Verification items for this drawing (mm, ordinates from the low corner). A direction names the side the tool comes from. Round coordinates to 2 decimals unless told otherwise and drop trailing zeros. Loops run counter-clockwise (first coordinate to the right, second up) from the corner with the lowest first, then second, coordinate; pieces in that order, holes last. Notation, with made-up numbers: M 52.25,18.25 L 74.25,18.25 A15 cw 74.25,45.25 Z; hole C -39.75,5.5 d3. An arc over 180 degrees is marked long. Use one line per item in the form item = value. Start each with the question number.
1. Go/stop test with flat-tipped pins: pin 1 (1 mm diameter, centred on x = 10.5, y = 68, fed in from -Z); pin 2 (4.5 mm diameter, centred on x = 16, y = 12.5, fed in from +Z); pin 3 (8 mm diameter, centred on x = 3.5, y = 33, fed in from -Z); pin 4 (8 mm diameter, centred on y = 22.5, z = 19, fed in from -X). Record where each tip stops, or that it passes through.
2. Cross-section at A-A (y = 13.3). Record the boundary of the cut face in (x, z).
3. Draft check along Y on the marked faces 1, 2, 3 and 4. Enter one of: pulls with the +Y half, pulls with the -Y half, needs draft (parallel to the pull), parting line crosses it, or undercut.
4. Cross-section at D-D (x = 2.5). Record the boundary of the cut face in (y, z), then the cut area to 3 significant figures.
5. Set-up check for the marked faces 5, 6 and 7: record each of +Z, -Z, +X, -X, +Y, -Y from which the full face is reachable in a straight line by a thin tool's end or side.
6. Material ranges on line 1 (Y direction, x = 15, z = 33); line 2 (Y direction, x = 15, z = 48); line 3 (X direction, y = 13, z = 9), recorded low to high.
7. Cross-section at B-B (x = 15). Record the boundary of the cut face in (y, z), then the cut area to 3 significant figures.
8. Cross-section at C-C (z = 7). Record the boundary of the cut face in (x, y), then the cut area to 3 significant figures.
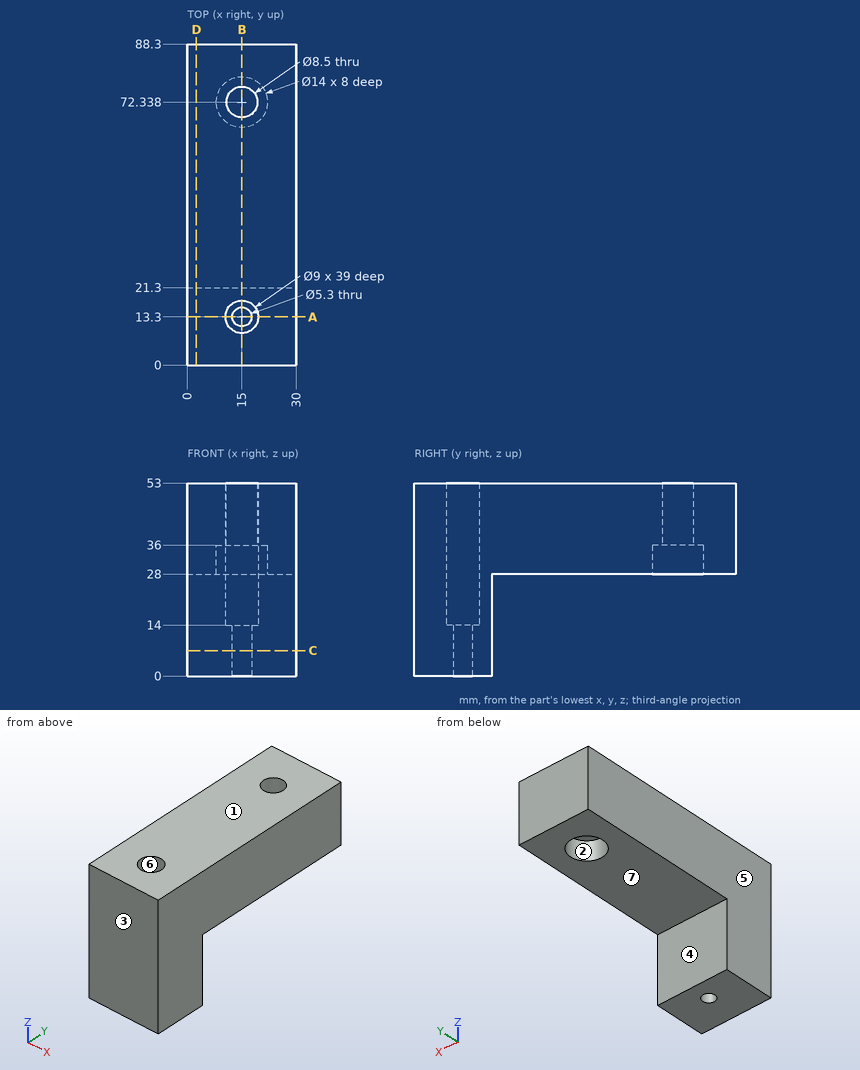
Reported:
q1.pin_1 = 36
q1.pin_2 = 14
q1.pin_3 = 28
q1.pin_4 = 0
q2.outline = M 0,0 L 12.35,0 L 12.35,14 L 10.5,14 L 10.5,53 L 0,53 Z; M 17.65,0 L 30,0 L 30,53 L 19.5,53 L 19.5,14 L 17.65,14 Z
q3.face_1 = needs draft
q3.face_2 = undercut
q3.face_3 = pulls with the -Y half
q3.face_4 = pulls with the +Y half
q4.outline = M 0,0 L 21.3,0 L 21.3,28 L 88.3,28 L 88.3,53 L 0,53 Z
q4.area = 2,800 mm²
q5.face_5 = +Z, -Z, -X, +Y, -Y
q5.face_6 = +Z
q5.face_7 = -Z, +X, -X, +Y
q6.line_1 = 0 to 8.8, 17.8 to 65.34, 79.34 to 88.3
q6.line_2 = 0 to 8.8, 17.8 to 68.09, 76.59 to 88.3
q6.line_3 = 0 to 12.37, 17.63 to 30
q7.outline = M 0,0 L 10.65,0 L 10.65,14 L 8.8,14 L 8.8,53 L 0,53 Z; M 15.95,0 L 21.3,0 L 21.3,28 L 65.34,28 L 65.34,36 L 68.09,36 L 68.09,53 L 17.8,53 L 17.8,14 L 15.95,14 Z; M 76.59,36 L 79.34,36 L 79.34,28 L 88.3,28 L 88.3,53 L 76.59,53 Z
q7.area = 2,120 mm²
q8.outline = M 0,0 L 30,0 L 30,21.3 L 0,21.3 Z; hole C 15,13.3 d5.3
q8.area = 617 mm²
